```python
from build123d import *

# Parameters (mm, degrees)
SKETCH_1_W          = 27.9
SKETCH_1_H          = 27.9
EXTRUDE_1_DEPTH     = 20
HOLE_WIZARD_M4_2_D  = 3.3
CUT_EXTRUDE_1_DEPTH = 46
CHAMFER_1_SIZE      = 3
HOLE_WIZARD_M4_3_D  = 3.3
HOLE_WIZARD_M4_4_D  = 3.3
FILLET_1_R          = 2
FILLET_2_R          = 3
CUT_EXTRUDE_2_DEPTH = 46
CUT_EXTRUDE_3_DEPTH = 46


with BuildPart() as part:
    # 草图1 → 凸台-拉伸1 (new, symmetric)
    with BuildSketch(Plane(origin=(0, 0, 0), x_dir=(1, 0, 0), z_dir=(0, 1, 0))):
        Rectangle(SKETCH_1_W, SKETCH_1_H)
    extrude(amount=EXTRUDE_1_DEPTH, both=True)

    # M4 螺纹孔2 (through all)
    with Locations(Plane(origin=(0, -20, 0), x_dir=(-1, 0, 0), z_dir=(0, -1, 0))):
        with Locations((8.95, -8.95), (8.95, 8.95), (-8.95, 8.95), (-8.95, -8.95)):
            Hole(HOLE_WIZARD_M4_2_D / 2)

    # 草图8 → 切除-拉伸1 (cut, symmetric)
    with BuildSketch(Plane.XZ.offset(20)):
        with BuildLine():
            ThreePointArc((-8.95, -5.45), (-6.475126266, -6.475126266), (-5.45, -8.95))
            Line((-5.45, -8.95), (5.45, -8.95))
            ThreePointArc((5.45, -8.95), (6.475126266, -6.475126266), (8.95, -5.45))
            Line((8.95, -5.45), (8.95, 5.45))
            ThreePointArc((8.95, 5.45), (6.475126266, 6.475126266), (5.45, 8.95))
            Line((5.45, 8.95), (-5.45, 8.95))
            ThreePointArc((-5.45, 8.95), (-6.475126266, 6.475126266), (-8.95, 5.45))
            Line((-8.95, 5.45), (-8.95, -5.45))
        make_face()
    extrude(amount=CUT_EXTRUDE_1_DEPTH, both=True, mode=Mode.SUBTRACT)

    # 倒角1
    chamfer_1_edges = [part.edges().sort_by_distance(p)[0] for p in [
        (13.95, 0, 13.95),
        (-13.95, 0, 13.95),
        (-13.95, 0, -13.95),
        (13.95, 0, -13.95),
    ]]
    chamfer(chamfer_1_edges, length=CHAMFER_1_SIZE)

    # M4 螺纹孔3 (through all)
    with Locations(Plane.ZY.offset(13.95)):
        with Locations((0, 16), (0, -16)):
            Hole(HOLE_WIZARD_M4_3_D / 2)

    # M4 螺纹孔4 (through all)
    with Locations(Plane.XY.offset(13.95)):
        with Locations((0, 16), (0, -16)):
            Hole(HOLE_WIZARD_M4_4_D / 2)

    # 圆角1
    fillet_1_edges = [part.edges().sort_by_distance(p)[0] for p in [
        (-13.95, 0, 10.95),
        (-13.95, 0, -10.95),
        (13.95, 0, -10.95),
        (13.95, 0, 10.95),
        (-10.95, 0, 13.95),
        (10.95, 0, 13.95),
        (-10.95, 0, -13.95),
        (10.95, 0, -13.95),
    ]]
    fillet(fillet_1_edges, radius=FILLET_1_R)

    # 圆角2
    fillet_2_edges = [part.edges().sort_by_distance(p)[0] for p in [
        (-8.95, 0, 5.45),
        (-5.45, 0, 8.95),
        (5.45, 0, 8.95),
        (8.95, 0, 5.45),
        (8.95, 0, -5.45),
        (5.45, 0, -8.95),
        (-5.45, 0, -8.95),
        (-8.95, 0, -5.45),
    ]]
    fillet(fillet_2_edges, radius=FILLET_2_R)

    # 草图15 → 切除-拉伸2 (cut, symmetric)
    with BuildSketch(Plane.ZY.offset(13.95)):
        with BuildLine():
            Line((-3.183718703, -9), (-3.183718703, 9))
            ThreePointArc((-3.183718703, 9), (0, 12.183718703), (3.183718703, 9))
            Line((3.183718703, 9), (3.183718703, -9))
            ThreePointArc((3.183718703, -9), (0, -12.183718703), (-3.183718703, -9))
        make_face()
    extrude(amount=CUT_EXTRUDE_2_DEPTH, both=True, mode=Mode.SUBTRACT)

    # 草图16 → 切除-拉伸3 (cut, symmetric)
    with BuildSketch(Plane(origin=(0, 0, -13.95), x_dir=(-1, 0, 0), z_dir=(0, 0, -1))):
        with BuildLine():
            Line((-3.183718703, -9), (-3.183718703, 9))
            ThreePointArc((-3.183718703, 9), (0, 12.183718703), (3.183718703, 9))
            Line((3.183718703, 9), (3.183718703, -9))
            ThreePointArc((3.183718703, -9), (0, -12.183718703), (-3.183718703, -9))
        make_face()
    extrude(amount=CUT_EXTRUDE_3_DEPTH, both=True, mode=Mode.SUBTRACT)


solid = part.part
```
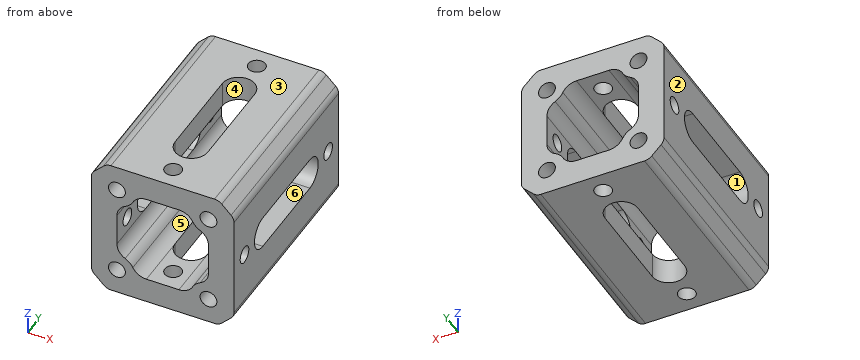
Model file for the job. Use its own axes, mm. Face numbers are marked on the shaded views. A direction names the side the tool comes from. Coordinates: 2 decimals unless noted, no trailing zeros. Write each loop counter-clockwise with the first axis right and the second up, starting at its lowest first coordinate (ties: lowest second). Pieces come first, ordered by that corner, then holes. Notation, with made-up numbers: (70.5, 35) - (84.5, 35) arc R13 ccw to (84.5, 59) - close; hole circle Ø10 at (61.25, 73). An arc over 180 degrees is marked (long way). Use a Markdown table: item, result. Add a question column.
Item 1: Two-plate mould, pull along Z, no slides. Class the marked faces 1, 2 and 3: pulls with the +Z half, pulls with the -Z half, needs draft (parallel to the pull), parting line crosses it, or undercut.
Item 2: Drill centre lines: line 1 along Y through (x, z) = (0, -11.6); line 2 along Z through (x, y) = (8, -11); line 3 along X through (y, z) = (7.5, 10). Where is each one in solid material? Low to high.
Item 3: Band-saw the part on A-A, the plane x = -1. Give the number of separate pieces and of enclosed holes in the cut face, and give its area (3 significant figures).
Item 4: 3-axis set-ups, long thin cutter, end or side, ignore diameter. For the marked faces 4, 5 and 6: which of +Z, -Z, +X, -X, +Y, -Y reach the whole face in a straight line?
Item 5: Band-saw the part on B-B, the plane z = 5.25. Write the cut outline in (x, y).
Item 6: Drop flat-ended pins along their axis: pin 1 (2.5 mm diameter, centred on y = 3.5, z = 12, fed in from +X); pin 2 (1.5 mm diameter, centred on x = 12.5, y = -3, fed in from -Z). Give the stop position or say it passes through.
A:
| question | item | result |
|---|---|---|
| 1 | face 1 | undercut |
| 1 | face 2 | needs draft |
| 1 | face 3 | pulls with the +Z half |
| 2 | line 1 | y = -20 to -17.65, -14.35 to -12.18, 12.18 to 14.35, 17.65 to 20 |
| 2 | line 2 | z = -13.95 to -10.3, -7.6 to -5.37, 5.37 to 7.6, 10.3 to 13.95 |
| 2 | line 3 | x = -13.95 to -10.22, -7.68 to -3.18, 3.18 to 7.68, 10.22 to 13.95 |
| 3 | separate pieces | 8 |
| 3 | enclosed holes | 0 |
| 3 | area | 107 mm² |
| 4 | face 4 | +Z, -Z |
| 4 | face 5 | +Y, -Y |
| 4 | face 6 | +X, -X |
| 5 | outline | (-13.95, -20) - (-8.12, -20) - (-8.12, 20) - (-13.95, 20) - close; (8.12, -20) - (13.95, -20) - (13.95, 20) - (8.12, 20) - close |
| 6 | pin 1 | stops at x = 13.85 |
| 6 | pin 2 | stops at z = -13.15 |
